Read the model definition and answer for the solid it produces. Units are mm, in the model's axes. A direction names the side the tool comes from. Round coordinates to 2 decimals unless told otherwise and drop trailing zeros. Write each loop counter-clockwise with the first axis right and the second up, starting at its lowest first coordinate (ties: lowest second). Pieces come first, ordered by that corner, then holes. Notation, with made-up numbers: (2, 18.25) - (14, 18.25) arc R28 cw to (14, 40.25) - close; hole circle Ø6 at (-24, -20). An arc over 180 degrees is marked (long way). One line per item, written item: value. Start each with the question number.
(1) Flat-ended cylindrical pins translate along their axes: pin 1 Ø2 at (x, z) = (0.5, 14) entering from +Y (3 decimals); pin 2 Ø1.2 at (y, z) = (0.5, 33) entering from -X (3 decimals); pin 3 Ø1 at (x, z) = (-0.5, 14.5) entering from -Y (3 decimals). Find the tip coordinate at first contact, or state that the pin passes through.
(2) A cutting plane is placed at D-D, the plane y = 0. Determine the outline of the cut face in (x, z) (3 decimals), plus the area to 3 significant figures.
(3) A cutting plane is placed at A-A, the plane x = 5.5. Determine the outline of the cut face in (y, z), plus the area to 3 significant figures.
(4) Find the intervals of material crossed by L1, parallel to Y at x = 0, z = 19.5 (3 decimals); L2, parallel to X at y = -0.25, z = 35 (3 decimals); L3, parallel to Y at x = -4.75, z = 43, in increasing order.
(5) For faces 1 (the face through (-4, -6.35, 25)), 2 (the face through (1.988, 5, 25)), 3 (the face through (5, -1.988, 25)), 4 (the face through (1.988, -5, 25)), 5 (the face through (-2.975, 0, 25)), determine the directions among +Z, -Z, +X, -X, +Y, -Y from which every point of the face is accessible in a straight line to the end or side of a thin tool.
(6) The mould has two halves that part along Y. Classify faces 6 (the face through (-5, 1.988, 25)), 7 (the face through (-6.35, -4, 25)), 8 (the face through (0, -2.975, 25)): +Y half, -Y half, draft (parallel to the pull), parting line (faces both ways), or undercut.
from build123d import *

# Parameters (mm, degrees)
F1_DEPTH = 50.8
F2_R     = 2
F3_DEPTH = 50


with BuildPart() as f1:
    # F0 (on Top) → F1 (new body)
    with BuildSketch(Plane.XY):
        Polygon((-1.9875, 6.35), (-6.35, 6.35), (-6.35, 1.9875), (-2.975, 1.9875), (-2.975, -1.9875), (-6.35, -1.9875), (-6.35, -6.35), (-1.9875, -6.35), (-1.9875, -2.975), (1.9875, -2.975), (1.9875, -6.35), (6.35, -6.35), (6.35, -1.9875), (2.975, -1.9875), (2.975, 1.9875), (6.35, 1.9875), (6.35, 6.35), (1.9875, 6.35), (1.9875, 2.975), (-1.9875, 2.975), align=None)
    extrude(amount=F1_DEPTH)

    # F2 (on face) → F3 (cut)
    with BuildSketch(Plane.XY.offset(50.8)):
        Circle(F2_R)
    extrude(amount=-F3_DEPTH, mode=Mode.SUBTRACT)


solid = f1.part
Here are the results:
1. pin 1: y = 2.975
1. pin 2: x = -2.975
1. pin 3: y = -2.975
2. outline: (-2.975, 0) - (2.975, 0) - (2.975, 50.8) - (2, 50.8) - (2, 0.8) - (-2, 0.8) - (-2, 50.8) - (-2.975, 50.8) - close
2. area: 102 mm²
3. outline: (-6.35, 0) - (-1.99, 0) - (-1.99, 50.8) - (-6.35, 50.8) - close; (1.99, 0) - (6.35, 0) - (6.35, 50.8) - (1.99, 50.8) - close
3. area: 443 mm²
4. L1: -2.975 to -2, 2 to 2.975
4. L2: -2.975 to -1.984, 1.984 to 2.975
4. L3: -6.35 to -1.99, 1.99 to 6.35
5. face 1: +Z, -Z, +X, -X, -Y
5. face 2: +Z, -Z, +Y
5. face 3: +Z, -Z, +X
5. face 4: +Z, -Z, -Y
5. face 5: +Z, -Z, -X
6. face 6: undercut
6. face 7: draft
6. face 8: -Y half
